Design review of the part built by this model. Coordinates are the model's own, in mm. Face numbers are marked on the shaded views. A direction names the side the tool comes from. Coordinates: 2 decimals unless noted, no trailing zeros. Write each loop counter-clockwise with the first axis right and the second up, starting at its lowest first coordinate (ties: lowest second). Pieces come first, ordered by that corner, then holes.
Q1. Insertion check: pin 1 (1.4 mm diameter, centred on x = 5.5, z = -2, fed in from +Y); pin 2 (2.5 mm diameter, centred on x = 0, z = 0, fed in from -Y); pin 3 (4 mm diameter, centred on x = 4, z = 2, fed in from +Y); pin 4 (1.5 mm diameter, centred on y = -0.5, z = 1.5, fed in from -X). Each pin has a flat end and moves straight along its axis. Give the tip position at first contact, or say it passes through.
Q2. For probe 1 along X at (y, z) = (-0.5, -2.75); probe 2 along Z at (x, y) = (1.5, -4); probe 3 along X at (y, z) = (-5.5, 0.5), list the stretches that pass through material, from the lowest coordinate up.
Q3. Take a section at C-C (z = -5.75). Give the boundary of the cut face in (x, y), and give its area (3 significant figures).
Q4. Mouldability with a two-part tool opening along Z and no side actions: class the marked faces 4, 5 and 6 as pulls with the +Z half, pulls with the -Z half, needs draft (parallel to the pull), parting line crosses it, or undercut.
Q5. Take a section at B-B (z = 0). Give the boundary of the cut face in (x, y), and give its area (3 significant figures).
Q6. Take a section at A-A (x = 0). Give the boundary of the cut face in (y, z).
Q7. Machinability: for the marked faces 1, 2 and 3, which of the approach directions +Z, -Z, +X, -X, +Y, -Y give a long, thin tool a straight path to every point of the face, cutting with its end or side? Answer none if there is none.
Q8. Take a section at D-D (y = -1.75). Give the boundary of the cut face in (x, z).
```python
from build123d import *

# Parameters (mm, degrees)
EXTRUDE_1_DEPTH   = 7.5
HOLE_WIZARD_M41_D = 3.3


with BuildPart() as part:
    # Эскиз1 → Бобышка-Вытянуть1 (new body, symmetric)
    with BuildSketch(Plane.XY):
        Polygon((4, 0), (-4, 0), (-4, -1.4), (-6.7, -1.4), (-6.7, -3.625153657), (-2.948598936, -6.2), (2.948598936, -6.2), (6.7, -3.625153657), (6.7, -1.4), (4, -1.4), align=None)
    extrude(amount=EXTRUDE_1_DEPTH, both=True)

    # Отверстие обработанное метчиком M41 (through all)
    with Locations(Plane.ZX):
        with Locations((0, 0)):
            Hole(HOLE_WIZARD_M41_D / 2)


solid = part.part
```
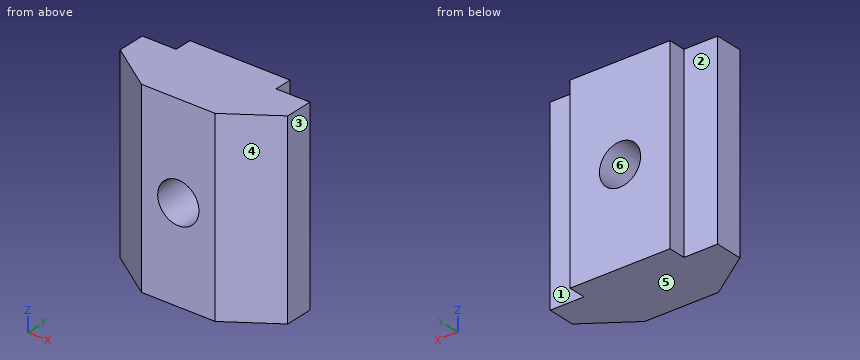
Response:
1. pin 1: stops at y = -1.4
1. pin 2: passes through
1. pin 3: stops at y = 0
1. pin 4: stops at x = -4
2. probe 1: x = -4 to 4
2. probe 2: z = -7.5 to -0.69, 0.69 to 7.5
2. probe 3: x = -3.97 to -1.57, 1.57 to 3.97
3. outline: (-6.7, -3.63) - (-2.95, -6.2) - (2.95, -6.2) - (6.7, -3.63) - (6.7, -1.4) - (4, -1.4) - (4, 0) - (-4, 0) - (-4, -1.4) - (-6.7, -1.4) - close
3. area: 65.9 mm2
4. face 4: needs draft
4. face 5: pulls with the -Z half
4. face 6: undercut
5. outline: (-6.7, -3.63) - (-2.95, -6.2) - (-1.65, -6.2) - (-1.65, 0) - (-4, 0) - (-4, -1.4) - (-6.7, -1.4) - close; (1.65, -6.2) - (2.95, -6.2) - (6.7, -3.63) - (6.7, -1.4) - (4, -1.4) - (4, 0) - (1.65, 0) - close
5. area: 45.4 mm2
6. outline: (-6.2, -7.5) - (0, -7.5) - (0, -1.65) - (-6.2, -1.65) - close; (-6.2, 1.65) - (0, 1.65) - (0, 7.5) - (-6.2, 7.5) - close
7. face 1: +Z, -Z, +X, +Y
7. face 2: +Z, -Z, -X, +Y
7. face 3: +Z, -Z, +X, +Y, -Y
8. outline: (-6.7, -7.5) - (6.7, -7.5) - (6.7, 7.5) - (-6.7, 7.5) - close; hole circle Ø3.3 at (0, 0)
